The listing builds one solid part. Answer for the finished solid, in the listing's coordinates (mm). A direction names the side the tool comes from. Give positions to 0.01 mm unless a question says otherwise; leave off trailing zeros. Order: outer loops, then holes, each group sorted by start corner. A loop starts at its lowest first (then second) coordinate and runs counter-clockwise, first axis right, second up.
```python
from build123d import *

# Parameters (mm, degrees)
SKETCH1_W           = 10
SKETCH1_H           = 10
SKETCH1_W_2         = 8
SKETCH1_H_2         = 8
BOSS_EXTRUDE1_DEPTH = 6
BOSS_EXTRUDE2_REACH = 11
SKETCH2_W           = 8
SKETCH2_H           = 1
SKETCH3_R           = 1.5
BOSS_EXTRUDE3_DEPTH = 1
BOSS_EXTRUDE4_DEPTH = 5
SKETCH5_R           = 0.75
CUT_EXTRUDE2_DEPTH  = 1


with BuildPart() as part:
    # Sketch1 → Boss-Extrude1 (new body)
    with BuildSketch(Plane(origin=(0, 0, 0), x_dir=(1, 0, 0), z_dir=(0, 1, 0))):
        with Locations((5, 5)):
            Rectangle(SKETCH1_W, SKETCH1_H)
        with Locations((5, 5)):
            Rectangle(SKETCH1_W_2, SKETCH1_H_2, mode=Mode.SUBTRACT)
    extrude(amount=BOSS_EXTRUDE1_DEPTH)

    # Sketch2 → Boss-Extrude2 (add, up to next)
    with BuildSketch(Plane.XY.offset(-9), mode=Mode.PRIVATE) as boss_extrude2_sk1:
        with Locations((5, 5.5)):
            Rectangle(SKETCH2_W, SKETCH2_H)
    boss_extrude2_tool1 = extrude(boss_extrude2_sk1.sketch, amount=BOSS_EXTRUDE2_REACH, mode=Mode.PRIVATE) - part.part
    add(boss_extrude2_tool1.solids().sort_by_distance((5, 5.5, -9))[0])

    # Sketch3 → Boss-Extrude3 (add)
    with BuildSketch(Plane(origin=(0, 6, 0), x_dir=(1, 0, 0), z_dir=(0, 1, 0))):
        with Locations((2.5, 2.5)):
            Circle(SKETCH3_R)
        with Locations((7.5, 2.5)):
            Circle(SKETCH3_R)
        with Locations((7.5, 7.5)):
            Circle(SKETCH3_R)
        with Locations((2.5, 7.5)):
            Circle(SKETCH3_R)
    extrude(amount=BOSS_EXTRUDE3_DEPTH)

    # Sketch4 → Boss-Extrude4 (add)
    with BuildSketch(Plane(origin=(0, 5, 0), x_dir=(-1, 0, 0), z_dir=(0, -1, 0))):
        with BuildLine():
            Line((-3.5, 5), (-2.964466094, 5))
            ThreePointArc((-2.964466094, 5), (-3.560660172, 6.439339828), (-5, 7.035533906))
            Line((-5, 7.035533906), (-5, 6.5))
            ThreePointArc((-5, 6.5), (-3.939339828, 6.060660172), (-3.5, 5))
        make_face()
        with BuildLine():
            Line((-5, 6.5), (-5, 7.035533906))
            ThreePointArc((-5, 7.035533906), (-5.778965109, 6.88058811), (-6.43933984, 6.439339817))
            ThreePointArc((-6.43933984, 6.439339817), (-6.880588116, 5.778965094), (-7.035533906, 5))
            Line((-7.035533906, 5), (-6.5, 5))
            ThreePointArc((-6.5, 5), (-6.060660172, 6.060660172), (-5, 6.5))
        make_face()
        with BuildLine():
            ThreePointArc((-5, 2.964466094), (-3.560660172, 3.560660172), (-2.964466094, 5))
            Line((-2.964466094, 5), (-3.5, 5))
            ThreePointArc((-3.5, 5), (-3.939339828, 3.939339828), (-5, 3.5))
            Line((-5, 3.5), (-5, 2.964466094))
        make_face()
        with BuildLine():
            ThreePointArc((-7.035533906, 5), (-6.439339828, 3.560660172), (-5, 2.964466094))
            Line((-5, 2.964466094), (-5, 3.5))
            ThreePointArc((-5, 3.5), (-6.060660172, 3.939339828), (-6.5, 5))
            Line((-6.5, 5), (-7.035533906, 5))
        make_face()
    extrude(amount=BOSS_EXTRUDE4_DEPTH)

    # Sketch5 → Cut-Extrude2 (cut)
    with BuildSketch(Plane(origin=(0, 5, 0), x_dir=(-1, 0, 0), z_dir=(0, -1, 0))):
        with BuildLine():
            ThreePointArc((-7.5, 6.75), (-6.969669914, 6.969669914), (-6.75, 7.5))
            Line((-6.75, 7.5), (-7.5, 7.5))
            Line((-7.5, 7.5), (-7.5, 6.75))
        make_face()
        with BuildLine():
            Line((-7.5, 7.5), (-6.75, 7.5))
            ThreePointArc((-6.75, 7.5), (-8.030330086, 8.030330086), (-7.5, 6.75))
            Line((-7.5, 6.75), (-7.5, 7.5))
        make_face()
        with Locations((-2.5, 7.5)):
            Circle(SKETCH5_R)
        with Locations((-2.5, 2.5)):
            Circle(SKETCH5_R)
        with Locations((-7.5, 2.5)):
            Circle(SKETCH5_R)
    extrude(amount=-CUT_EXTRUDE2_DEPTH, mode=Mode.SUBTRACT)


solid = part.part
```
1) Given P1, Ø1.4, axis at x = 7.5, z = -7.5, coming from the -Y side; P2, Ø3, axis at x = 4.5, z = -5.5, coming from the -Y side; P3, Ø2.5, axis at x = 7.5, z = -2.5, coming from the -Y side; P4, Ø1, axis at x = 9, z = -9, coming from the +Y side, each flat-ended and moving along its own axis, determine where each tip first touches the part or whether it passes through.
Geometry says:
P1: stops at y = 6
P2: stops at y = 0
P3: stops at y = 5
P4: stops at y = 6
2) Find section B-B (y = 5.5). Write down the section's boundary in (x, z).
Geometry says:
outline: (0, -10) - (10, -10) - (10, 0) - (0, 0) - close; hole circle Ø1.5 at (2.5, -7.5); hole circle Ø1.5 at (2.5, -2.5); hole circle Ø1.5 at (7.5, -7.5); hole circle Ø1.5 at (7.5, -2.5)
3) Find section C-C (x = 2.5). Write down the section's boundary in (y, z), then the cut area to 3 significant figures.
Geometry says:
outline: (0, -10) - (6, -10) - (6, -9) - (7, -9) - (7, -6) - (6, -6) - (6, -4) - (7, -4) - (7, -1) - (6, -1) - (6, 0) - (0, 0) - (0, -1) - (5, -1) - (5, -1.75) - (6, -1.75) - (6, -3.25) - (5, -3.25) - (5, -6.75) - (6, -6.75) - (6, -8.25) - (5, -8.25) - (5, -9) - (0, -9) - close
area: 23.0 mm2
4) For a pull along Z with two mould halves and no side action, classify faces 4 (the cylindrical face through (2.175, 6.493, -1.036)), 5 (the flat face through (10, 3, -5)) as +Z half, -Z half, draft (parallel to the pull), parting line (faces both ways), or undercut.
Geometry says:
face 4: undercut
face 5: draft
5) Straight lines are drawn through the part: probe 1 along X at (y, z) = (5.65, -2.5); probe 2 along Z at (x, y) = (2.5, 5.8); probe 3 along Z at (x, y) = (5, 4). For each, find the intervals that lie inside material, in ascending order.
Geometry says:
probe 1: x = 0 to 1.75, 3.25 to 6.75, 8.25 to 10
probe 2: z = -10 to -8.25, -6.75 to -3.25, -1.75 to 0
probe 3: z = -10 to -9, -7.04 to -6.5, -3.5 to -2.96, -1 to 0
6) Find section D-D (z = -4.5). Write down the section's boundary in (x, y).
Geometry says:
outline: (0, 0) - (1, 0) - (1, 5) - (3.03, 5) - (3.03, 0) - (3.59, 0) - (3.59, 5) - (6.41, 5) - (6.41, 0) - (6.97, 0) - (6.97, 5) - (9, 5) - (9, 0) - (10, 0) - (10, 6) - (0, 6) - close
7) A tool of negligible diameter and unlimited length cuts with its end or side. For faces 1 (the cylindrical face through (6.3, 6.5, -1.6)), 2 (the flat face through (5, 5, -5)), 3 (the flat face through (0.5, 0, -5.1)), from which of +Z, -Z, +X, -X, +Y, -Y can it reach the whole face along a straight path? Write none if from no direction.
Geometry says:
face 1: +Y
face 2: -Y
face 3: +Z, -Z, +X, -X, -Y
8) Find section A-A (y = 2). Write down the section's boundary in (x, z).
Geometry says:
outline: (0, -10) - (10, -10) - (10, 0) - (0, 0) - close; circle Ø4.07 at (5, -5); hole (1, -9) - (9, -9) - (9, -1) - (1, -1) - close; hole circle Ø3 at (5, -5)
